Design review of the part built by this model. Coordinates are the model's own, in mm. A direction names the side the tool comes from. Coordinates: 2 decimals unless noted, no trailing zeros. Loops run counter-clockwise (first coordinate to the right, second up) from the corner with the lowest first, then second, coordinate; pieces in that order, holes last.
Q1. Draft analysis for pull direction Y (two halves, no side actions). For faces 3 (the face through (7.451, 52.716, -11.706)), 4 (the face through (5.42, -24.51, 43.82)), 5 (the face through (11, 11, -35)), state which applies: released by +Y, released by -Y, zero draft, split by the parting line, or undercut.
Q2. Add section C-C on z = 31. Give the boundary of the cut face in (x, y), and give its area (3 significant figures).
Q3. Machinability: for faces 1 (the face through (5.577, -24.331, -26.533)), 2 (the face through (4, 47, 29)), which of the approach directions +Z, -Z, +X, -X, +Y, -Y give a long, thin tool a straight path to every point of the face, cutting with its end or side? Answer none if there is none.
Q4. Add section A-A on y = 0. Give the boundary of the cut face in (x, z), and give its area (3 significant figures).
Q5. Wall thickness on probe 1 along Y at (x, z) = (8, 0); probe 2 along Y at (x, z) = (1, 38); probe 3 along Z at (x, y) = (0.5, -12): over which ranges is each line inside the solid? List them lowest first.
Q6. Add section D-D on y = -22.5. Give the boundary of the cut face in (x, z).
Q7. For P1, Ø12, axis at y = -22.5, z = 38.97, coming from the +X side; P2, Ø4, axis at x = 8.5, y = 36.5, coming from the -Z side; P3, Ø6, axis at x = 5, z = 49.5, coming from the -Y side; P4, Ø1, axis at x = 2.5, y = -40.5, coming from the -Z side, all flat-tipped, find the tip position at first contact; note any pin that passes through.
Q8. Add section B-B on x = 5.75. Give the boundary of the cut face in (y, z), and give its area (3 significant figures).
```python
from build123d import *

# Parameters (mm, degrees)
M10_CLEARANCE_HOLE1_D = 10.5


with BuildPart() as part:
    # Sketch1 → Revolve1 (revolve)
    with BuildSketch(Plane(origin=(0, 0, 0), x_dir=(1, 0, 0), z_dir=(0, 1, 0)), mode=Mode.PRIVATE) as revolve1_sk:
        Polygon((0, 54), (0, 36), (11, 36), (11, 54), (4, 54), (4, 64), (0, 64), align=None)
    revolve(revolve1_sk.sketch.rotate(Axis((-0.5, 0, 0), (1, 0, 0)), 180), axis=Axis((-0.5, 0, 0), (1, 0, 0)))

    # M10 Clearance Hole1 (through all)
    with Locations(Plane(origin=(11, 0, 0), x_dir=(0, 0, -1), z_dir=(1, 0, 0))):
        with Locations((-38.97114317, 22.5), (0, 45), (38.97114317, 22.5), (38.97114317, -22.5), (0, -45), (-38.97114317, -22.5)):
            Hole(M10_CLEARANCE_HOLE1_D / 2)


solid = part.part
```
Entries:
1. face 3: split by the parting line
1. face 4: undercut
1. face 5: zero draft
2. outline: (0, -55.99) - (4, -55.99) - (4, -44.22) - (11, -44.22) - (11, -18.3) - (0, -18.3) - close; (0, 18.3) - (11, 18.3) - (11, 44.22) - (4, 44.22) - (4, 55.99) - (0, 55.99) - close
2. area: 664 mm2
3. face 1: +X, -X
3. face 2: +X
4. outline: (0, -64) - (4, -64) - (4, -54) - (11, -54) - (11, -36) - (0, -36) - close; (0, 36) - (11, 36) - (11, 54) - (4, 54) - (4, 64) - (0, 64) - close
4. area: 476 mm2
5. probe 1: y = -54 to -50.25, -39.75 to -36, 36 to 39.75, 50.25 to 54
5. probe 2: y = -51.5 to -27.66, -17.34 to 17.34, 27.66 to 51.5
5. probe 3: z = -62.86 to -33.94, 33.94 to 62.86
6. outline: (0, -59.91) - (4, -59.91) - (4, -49.09) - (11, -49.09) - (11, -44.22) - (0, -44.22) - close; (0, -33.72) - (11, -33.72) - (11, -28.1) - (0, -28.1) - close; (0, 28.1) - (11, 28.1) - (11, 33.72) - (0, 33.72) - close; (0, 44.22) - (11, 44.22) - (11, 49.09) - (4, 49.09) - (4, 59.91) - (0, 59.91) - close
7. P1: stops at x = 11
7. P2: stops at z = -41.54
7. P3: stops at y = -43.79
7. P4: stops at z = -49.96
8. outline: circle Ø108 at (0, 0); hole circle Ø10.5 at (-45, 0); hole circle Ø72 at (0, 0); hole circle Ø10.5 at (-22.5, -38.97); hole circle Ø10.5 at (-22.5, 38.97); hole circle Ø10.5 at (22.5, -38.97); hole circle Ø10.5 at (22.5, 38.97); hole circle Ø10.5 at (45, 0)
8. area: 4,570 mm2
